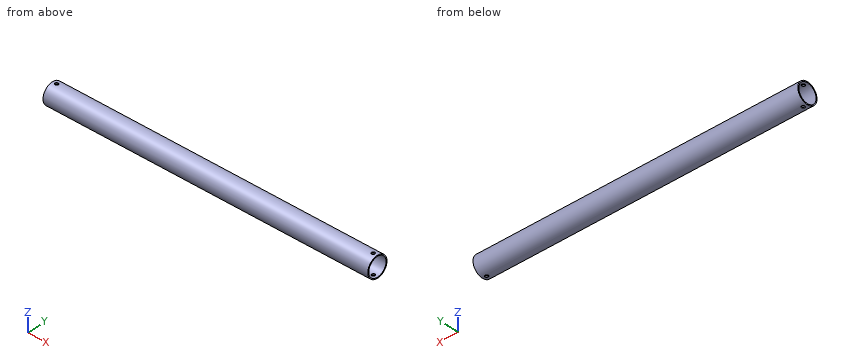
Autodesk Inventor part; units mm, degrees
ref_plane "Work Plane1" through (0, 0, 17.4625) normal (0, 0, 1) x (1, 0, 0)
ref_plane "YZ Plane" through (0, 0, 0) normal (1, 0, 0) x (0, 1, 0)
ref_plane "XZ Plane" through (0, 0, 0) normal (0, 1, 0) x (-1, 0, 0)
sketch "Sketch1" plane through (0, 0, 0) normal (1, 0, 0) x (0, 1, 0)
  circle A0 centre (0, 0) radius 15.875
  circle A1 centre (0, 0) radius 14.2875
  dimension "d0" = 31.75
  dimension "d2" = 1.5875
extrude "Extrusion1" add sketch "Sketch1" along normal mid plane 500.0625
ref_plane "Work Plane1" through (0, 0, 17.4625) normal (0, 0, 1) x (1, 0, 0)
sketch "Sketch3" plane through (0, 0, 17.4625) normal (0, 0, 1) x (1, 0, 0)
  line L0 (-250.0312, 15.875) -> (-250.0312, -15.875)
  line L1 (250.0312, -15.875) -> (250.0312, 15.875)
  point P0 (0, 0)
  point P1 (-243.6812, 0)
  point P2 (-250.0312, 0)
  point P3 (243.6812, 0)
  point P4 (250.0312, 0)
  dimension "d15" = 6.35
  dimension "d16" = 6.35
hole "Hole2" at (-243.6812, 0, 17.4625) at (243.6812, 0, 17.4625) direction (0, 0, -1) diameter 5.1054 end through all
properties part number "GI - 003" material "Polycarbonate, Smoke"
Here's how the part is built. I have some questions about the finished solid (model axes, mm). Coordinates: 2 decimals unless noted, no trailing zeros. Write each loop counter-clockwise with the first axis right and the second up, starting at its lowest first coordinate (ties: lowest second). Pieces come first, ordered by that corner, then holes. Notation, with made-up numbers: (86, -28.5) -> (99, -28.5) arc R10 ccw to (99, -24.5) -> close; hole circle Ø3 at (80.5, 26). An arc over 180 degrees is marked (long way). Use a Markdown table: item, result. Add a question column.
(1) I'm going to push flat-ended pins straight in: P1, Ø10, axis at x = -159.5, z = 8.5, coming from the -Y side; P2, Ø4, axis at x = 45.5, z = -5.5, coming from the +Y side; P3, Ø3, axis at x = -169.5, y = 10.5, coming from the -Z side. Where does each tip first touch, or does it pass through?
(2) If we section it at B-B, the plane y = 7: Write out the boundary of the cut face in (x, z).
(3) If we section it at A-A, the plane z = 0: Write out the boundary of the cut face in (x, y) (1 decimal), and give its area (3 significant figures).
(4) Please list where these lines run through material, in increasing order: line 1 (X direction, y = 0, z = 15); line 2 (Z direction, x = 15, y = 0) (1 decimal); line 3 (Z direction, x = 145.5, y = -1).
Outcome:
| question | item | result |
|---|---|---|
| 1 | P1 | stops at y = -15.48 |
| 1 | P2 | stops at y = 15.48 |
| 1 | P3 | stops at z = -13.08 |
| 2 | outline | (-250.03, -14.25) -> (250.03, -14.25) -> (250.03, -12.46) -> (-250.03, -12.46) -> close; (-250.03, 12.46) -> (250.03, 12.46) -> (250.03, 14.25) -> (-250.03, 14.25) -> close |
| 3 | outline | (-250, -15.9) -> (250, -15.9) -> (250, -14.3) -> (-250, -14.3) -> close; (-250, 14.3) -> (250, 14.3) -> (250, 15.9) -> (-250, 15.9) -> close |
| 3 | area | 1,590 mm^2 |
| 4 | line 1 | x = -250.03 to -246.23, -241.13 to 241.13, 246.23 to 250.03 |
| 4 | line 2 | z = -15.9 to -14.3, 14.3 to 15.9 |
| 4 | line 3 | z = -15.84 to -14.25, 14.25 to 15.84 |
